Drawing for the job (mm, zero at the part's lowest x, y, z). Round coordinates to 2 decimals unless told otherwise and drop trailing zeros. Loops run counter-clockwise (first coordinate to the right, second up) from the corner with the lowest first, then second, coordinate; pieces in that order, holes last. Notation, with made-up numbers: M 36.5,85 L 87.5,85 A16 cw 87.5,107 Z; hole C 57,38 d9. An arc over 180 degrees is marked long. Answer in a Markdown table with one row per item.
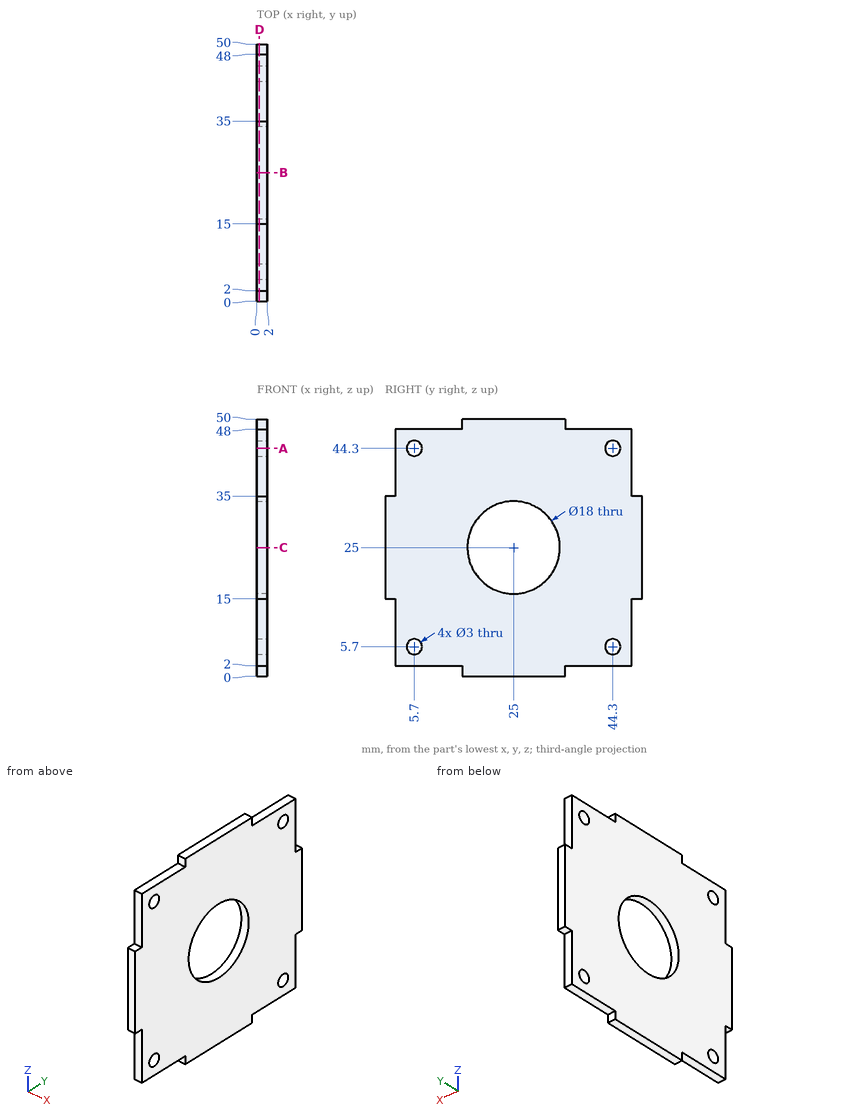
1. Saw through at B-B (y = 25). Write the cut outline in (x, z), and give its area (3 significant figures).
Verdict:
| item | result |
|---|---|
| outline | M 0,0 L 2,0 L 2,16 L 0,16 Z; M 0,34 L 2,34 L 2,50 L 0,50 Z |
| area | 64.0 mm² |
2. Pin check, flat tips, straight feed: pin 1 (1 mm diameter, centred on x = 1, z = 39.5, fed in from +Y); pin 2 (0.6 mm diameter, centred on x = 1, y = 6, fed in from -Z); pin 3 (1 mm diameter, centred on x = 1, y = 0.5, fed in from +Z). Stop position of each tip, or through.
Verdict:
| item | result |
|---|---|
| pin 1 | stops at y = 48 |
| pin 2 | stops at z = 2 |
| pin 3 | stops at z = 35 |
3. Wall check: probe 1 along Z at (x, y) = (0.7, 5.7); probe 2 along Y at (x, z) = (1, 25). Give the ranges that are in metal, low to high.
Verdict:
| item | result |
|---|---|
| probe 1 | z = 2 to 4.2, 7.2 to 42.8, 45.8 to 48 |
| probe 2 | y = 0 to 16, 34 to 50 |
4. Saw through at A-A (z = 44.3). Write the cut outline in (x, y).
Verdict:
| item | result |
|---|---|
| outline | M 0,2 L 2,2 L 2,4.2 L 0,4.2 Z; M 0,7.2 L 2,7.2 L 2,42.8 L 0,42.8 Z; M 0,45.8 L 2,45.8 L 2,48 L 0,48 Z |
5. Saw through at D-D (x = 0.5). Write the cut outline in (y, z), and give its area (3 significant figures).
Verdict:
| item | result |
|---|---|
| outline | M 0,15 L 2,15 L 2,2 L 15,2 L 15,0 L 35,0 L 35,2 L 48,2 L 48,15 L 50,15 L 50,35 L 48,35 L 48,48 L 35,48 L 35,50 L 15,50 L 15,48 L 2,48 L 2,35 L 0,35 Z; hole C 5.7,5.7 d3; hole C 5.7,44.3 d3; hole C 25,25 d18; hole C 44.3,5.7 d3; hole C 44.3,44.3 d3 |
| area | 1,990 mm² |
